Check sheet for the drawn part. Datum: minimum x, y, z corner. Units: mm. A direction names the side the tool comes from. Round coordinates to 2 decimals unless told otherwise and drop trailing zeros. Order: outer loops, then holes, each group sorted by start corner. A loop starts at its lowest first (then second) coordinate and runs counter-clockwise, first axis right, second up. Notation, with made-up numbers: (78.5, 28) -> (118.5, 28) arc R15 ccw to (118.5, 57) -> close; hole circle Ø4 at (82, 31.25). An arc over 180 degrees is marked (long way). Answer as a JSON object with one key per item and string values. Group by question number.
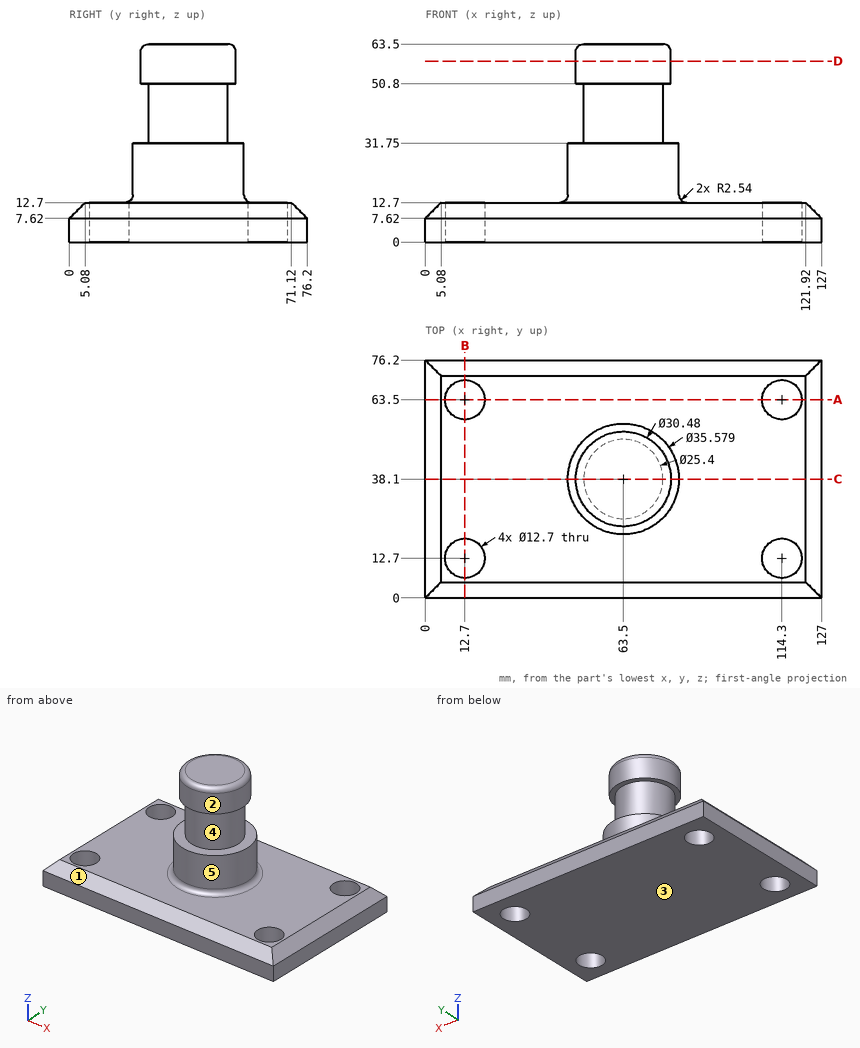
Item 1: Sectioned sample at D-D, the plane z = 58. Enter the section's corners in (x, y).
Item 2: Thickness scan on L1, parallel to Y at x = 12.7, z = 4.5; L2, parallel to Z at x = 92, y = 67.5; L3, parallel to Y at x = 63.5, z = 47.5. Record the ranges inside material, lowest first.
Item 3: Set-up check for the marked faces 1 and 2: record each of +Z, -Z, +X, -X, +Y, -Y from which the full face is reachable in a straight line by a thin tool's end or side.
Item 4: Sectioned sample at A-A, the plane y = 63.5. Enter the section's corners in (x, z).
Item 5: Mould release check, pull along Z, two halves, no side actions. Record for the marked faces 3, 4 and 5: pulls with the +Z half, pulls with the -Z half, needs draft (parallel to the pull), parting line crosses it, or undercut.
Item 6: Sectioned sample at C-C, the plane y = 38.1. Enter the section's corners in (x, z).
Item 7: Depth check by flat-ended pin: pin 1 Ø12 at (x, z) = (24, 16) entering from -Y; pin 2 Ø3 at (y, z) = (32, 42.5) entering from +X; pin 3 Ø2 at (x, z) = (59.5, 47) entering from -Y. Enter the tip coordinate at first touch or a pass-through.
Item 8: Sectioned sample at B-B, the plane x = 12.7. Enter the section's corners in (y, z), then the cut area to 3 significant figures.
Result:
{
 "1": {"outline": "circle Ø30.48 at (63.5, 38.1)"},
 "2": {"L1": "y = 0 to 6.35, 19.05 to 57.15, 69.85 to 76.2", "L2": "z = 0 to 12.7", "L3": "y = 25.4 to 50.8"},
 "3": {"face 1": "+Z, +X, -X, -Y", "face 2": "+Z"},
 "4": {"outline": "(0, 0) -> (6.35, 0) -> (6.35, 12.7) -> (5.08, 12.7) -> (0, 7.62) -> close; (19.05, 0) -> (107.95, 0) -> (107.95, 12.7) -> (19.05, 12.7) -> close; (120.65, 0) -> (127, 0) -> (127, 7.62) -> (121.92, 12.7) -> (120.65, 12.7) -> close"},
 "5": {"face 3": "pulls with the -Z half", "face 4": "undercut", "face 5": "needs draft"},
 "6": {"outline": "(0, 0) -> (127, 0) -> (127, 7.62) -> (121.92, 12.7) -> (83.83, 12.7) arc R2.54 cw to (81.29, 15.24) -> (81.29, 31.75) -> (76.2, 31.75) -> (76.2, 50.8) -> (78.74, 50.8) -> (78.74, 60.96) arc R2.54 ccw to (76.2, 63.5) -> (50.8, 63.5) arc R2.54 ccw to (48.26, 60.96) -> (48.26, 50.8) -> (50.8, 50.8) -> (50.8, 31.75) -> (45.71, 31.75) -> (45.71, 15.24) arc R2.54 cw to (43.17, 12.7) -> (5.08, 12.7) -> (0, 7.62) -> close"},
 "7": {"pin 1": "stops at y = 2.38", "pin 2": "stops at x = 75.34", "pin 3": "stops at y = 25.76"},
 "8": {"outline": "(0, 0) -> (6.35, 0) -> (6.35, 12.7) -> (5.08, 12.7) -> (0, 7.62) -> close; (19.05, 0) -> (57.15, 0) -> (57.15, 12.7) -> (19.05, 12.7) -> close; (69.85, 0) -> (76.2, 0) -> (76.2, 7.62) -> (71.12, 12.7) -> (69.85, 12.7) -> close", "area": "619 mm2"}
}
